For this review, take the finished solid that the model builds, in its own axes (mm). Face numbers are marked on the shaded views. A direction names the side the tool comes from. Give positions to 0.01 mm unless a question says otherwise; leave off trailing zeros. Loops run counter-clockwise (first coordinate to the right, second up) from the corner with the lowest first, then second, coordinate; pieces in that order, holes last. Notation, with made-up numbers: (10, -26) - (25, -26) arc R18 cw to (25, -8) - close; hole circle Ø5 at (62, -35.75). An arc over 180 degrees is marked (long way). Put each result on its own line as item: value.
Autodesk Inventor part; units mm, degrees
ref_plane "YZ Plane" through (0, 0, 0) normal (1, 0, 0) x (0, 1, 0)
ref_plane "XZ Plane" through (0, 0, 0) normal (0, 1, 0) x (-1, 0, 0)
ref_plane "XY Plane" through (0, 0, 0) normal (0, 0, 1) x (1, 0, 0)
sketch "Sketch1" plane through (0, 0, 0) normal (1, 0, 0) x (0, 1, 0)
  circle A0 centre (0, 0) radius 25.4
  circle A1 centre (0, 0) radius 4.445
  dimension "d3" = 8.89
extrude "Extrusion1" add sketch "Sketch1" along normal blind 25.4
sketch "Sketch2" plane through (0, 0, 0) normal (-1, 0, 0) x (0, 0, 1)
  circle A0 centre (0, 0) radius 10.9855
  dimension "d6" = 21.971
extrude "Extrusion2" cut sketch "Sketch2" against normal blind 6.858
sketch "Sketch3" plane through (25.4, 0, 0) normal (1, 0, 0) x (0, 0, -1)
  circle A0 centre (0, 0) radius 10.9855
  dimension "d9" = 21.971
extrude "Extrusion3" cut sketch "Sketch3" against normal blind 6.858
sketch "Sketch5" plane through (25.4, 0, 0) normal (1, 0, 0) x (0, 0, -1)
  circle A0 centre (0, 0) radius 4.445
  circle A1 centre (0, 0) radius 11.176
  dimension "d48" = 22.352
extrude "Extrusion8" cut sketch "Sketch5" against normal up to surface (6.858 mm away)
properties part number "correct_wheel"
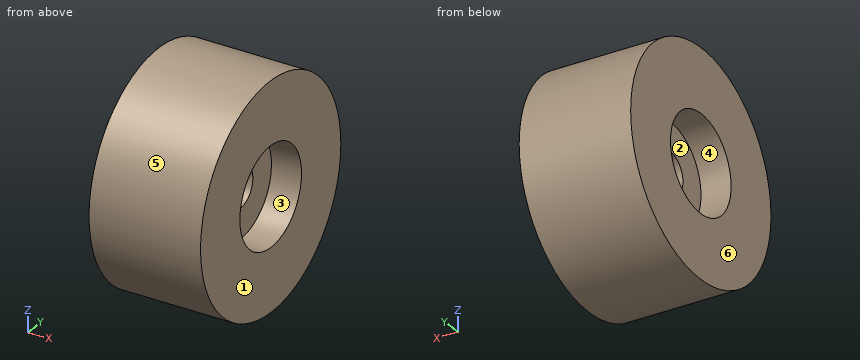
1) Take a section at D-D on z = -5.5. State the section outline as (x, y) points, and give its area (3 significant figures).
Geometry check:
outline: (0, -24.8) - (25.4, -24.8) - (25.4, -9.73) - (18.54, -9.73) - (18.54, 9.73) - (25.4, 9.73) - (25.4, 24.8) - (0, 24.8) - (0, 9.51) - (6.86, 9.51) - (6.86, -9.51) - (0, -9.51) - close
area: 996 mm²
2) Take a section at A-A on y = 0. State the section outline as (x, z) points (1 decimal).
Geometry check:
outline: (0, -25.4) - (25.4, -25.4) - (25.4, -11.2) - (18.5, -11.2) - (18.5, -4.4) - (6.9, -4.4) - (6.9, -11) - (0, -11) - close; (0, 11) - (6.9, 11) - (6.9, 4.4) - (18.5, 4.4) - (18.5, 11.2) - (25.4, 11.2) - (25.4, 25.4) - (0, 25.4) - close
3) For the marked faces 1, 2 and 3, list the 3-axis set-ups (+Z, -Z, +X, -X, +Y, -Y) from which the entire face can be reached by the end or side of a thin tool; tool diameter is ignored.
Geometry check:
face 1: +Z, -Z, +X, +Y, -Y
face 2: -X
face 3: +X
4) Draft analysis for pull direction Y (two halves, no side actions). For the marked faces 4, 5 and 6, state which applies: pulls with the +Y half, pulls with the -Y half, needs draft (parallel to the pull), parting line crosses it, or undercut.
Geometry check:
face 4: undercut
face 5: parting line crosses it
face 6: needs draft
5) Take a section at C-C on x = 2.5. State the section outline as (y, z) points.
Geometry check:
outline: circle Ø50.8 at (0, 0); hole circle Ø21.97 at (0, 0)
6) Wall thickness on line 1 (X direction, y = 4, z = -3); line 2 (Z direction, x = 11, y = 0) (3 decimals); line 3 (Y direction, x = 16, z = -1): over which ranges is each line inside the solid? List them lowest first.
Geometry check:
line 1: x = 6.86 to 18.54
line 2: z = -25.4 to -4.445, 4.445 to 25.4
line 3: y = -25.38 to -4.33, 4.33 to 25.38
7) Insertion check: pin 1 Ø20 at (y, z) = (0, 0) entering from -X; pin 2 Ø2 at (x, z) = (7.5, -1.5) entering from -Y; pin 3 Ø3 at (x, z) = (2.5, -4) entering from +Y; pin 4 Ø24.5 at (y, z) = (-3, 3) entering from +X. Each pin has a flat end and moves straight along its axis. Give the tip position at first contact, or say it passes through.
Geometry check:
pin 1: stops at x = 6.86
pin 2: stops at y = -25.4
pin 3: stops at y = 25.28
pin 4: stops at x = 25.4
